Geometry check sheet. Reference: the model listing, model coordinates, mm. Face numbers are marked on the shaded views. A direction names the side the tool comes from. Coordinates: 2 decimals unless noted, no trailing zeros. Write each loop counter-clockwise with the first axis right and the second up, starting at its lowest first coordinate (ties: lowest second). Pieces come first, ordered by that corner, then holes. Notation, with made-up numbers: M 50.25,11 L 106.25,11 A20 cw 106.25,35 Z; hole C -29,72.25 d4. An arc over 180 degrees is marked long. Write each question's results on one line, items separated by ' | '.
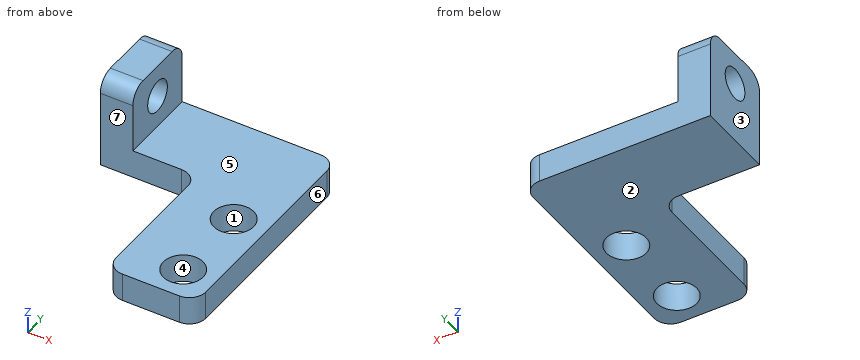
Autodesk Inventor part; units mm, degrees
ref_plane "YZ Plane" through (0, 0, 0) normal (1, 0, 0) x (0, 1, 0)
ref_plane "XZ Plane" through (0, 0, 0) normal (0, 1, 0) x (-1, 0, 0)
ref_plane "XY Plane" through (0, 0, 0) normal (0, 0, 1) x (1, 0, 0)
ref_plane "Work Plane1" through (0, 0, 0) normal (0, 0, 1) x (1, 0, 0)
sketch "Sketch1" plane through (0, 0, 0) normal (0, 0, 1) x (1, 0, 0)
  circle A0 centre (-18.4345, 53.6439) radius 1.95
  circle A1 centre (-18.4345, 43.6439) radius 1.95
  circle A2 centre (-45.5, -14.5) radius 2.1
  circle A3 centre (-14.5, -14.5) radius 2.1
  circle A4 centre (-14.5, 16.5) radius 2.1
  circle A5 centre (-45.5, 16.5) radius 2.1
  circle A6 centre (-30, 1) radius 13
  arc A7 (30, -41.6762) -> (-30, -41.6762) centre (0, -65) ccw
  line L0 (30, -41.6762) -> (30, -22)
  line L1 (30, -22) -> (10.1716, -22)
  line L2 (10.1716, -22) -> (7, -18.8284)
  line L3 (7, -18.8284) -> (7, 20.8284)
  line L4 (7, 20.8284) -> (10.1716, 24)
  line L5 (10.1716, 24) -> (26, 24)
  line L6 (26, 70.5) -> (26, 24)
  arc A8 (26, 70.5) -> (5.5, 91) centre (5.5, 70.5) ccw
  line L7 (-5.5, 91) -> (5.5, 91)
  arc A9 (-5.5, 91) -> (-26, 70.5) centre (-5.5, 70.5) ccw
  line L8 (-26, 24) -> (-26, 70.5)
  line L9 (-26, 24) -> (-49.8284, 24)
  line L10 (-49.8284, 24) -> (-53, 20.8284)
  line L11 (-53, 20.8284) -> (-53, -18.8284)
  line L12 (-53, -18.8284) -> (-49.8284, -22)
  line L13 (-49.8284, -22) -> (-30, -22)
  line L14 (-30, -22) -> (-30, -41.6762)
  circle A10 centre (18.4345, 43.6439) radius 1.95
  circle A11 centre (18.4345, 53.6439) radius 1.95
  line L15 (11.4345, 57.6439) -> (22.4345, 57.6439)
  line L16 (22.4345, 57.6439) -> (22.4345, 39.6439)
  line L17 (22.4345, 39.6439) -> (11.4345, 39.6439)
  line L18 (11.4345, 39.6439) -> (11.4345, 57.6439)
  circle A12 centre (18.4345, 53.6439) radius 2.45
  circle A13 centre (18.4345, 43.6439) radius 2.45
  line L19 (11.4345, 39.6439) -> (11.4345, 57.6439)
  line L20 (11.4345, 57.6439) -> (22.4345, 57.6439)
  line L21 (22.4345, 57.6439) -> (22.4345, 67.6439)
  line L22 (22.4345, 67.6439) -> (11.4345, 67.6439)
  line L23 (11.4345, 67.6439) -> (11.4345, 57.6439)
  line L24 (9.2719, 63.6439) -> (5.8371, 63.6439)
  line L25 (11.4345, 67.6439) -> (-0.5655, 67.6439)
  line L26 (-0.5655, 67.6439) -> (-0.5655, 57.8782)
  line L27 (-0.5655, 57.8782) -> (11.4345, 57.8782)
  line L28 (11.4345, 57.8782) -> (11.4345, 67.6439)
  point P0 (0, 0)
  point P1 (11.4345, 48.6439)
  dimension "d0" = 4
  dimension "d1" = 4
  dimension "d2" = 4
  dimension "d3" = 7
  dimension "d13" = 0.5
  dimension "d14" = 0.5
  dimension "d27" = 15
  dimension "d28" = 4
  dimension "d29" = 11
  dimension "d30" = 12
  dimension "d31" = 90
  dimension "d32" = 79.8782
  dimension "d33" = 61.6439
  dimension "d34" = 20.7281
  dimension "d35" = 24.1629
extrude "Extrusion1" add sketch "Sketch1" along normal blind 3.5 contours L23 L22 L21 L15 | L15 L16 L17 L18 | L27 L26 L25 L23
sketch "Sketch3" plane through (0, 0, 3.5) normal (0, 0, 1) x (1, 0, 0)
  circle A0 centre (18.4345, 43.6439) radius 2.45
  circle A1 centre (18.4345, 53.6439) radius 2.45
  line L0 (11.4345, 39.6439) -> (22.4345, 39.6439)
  line L1 (22.4345, 39.6439) -> (22.4345, 67.6439)
  line L2 (22.4345, 67.6439) -> (-0.5655, 67.6439)
  line L3 (-0.5655, 67.6439) -> (-0.5655, 57.8782)
  line L4 (-0.5655, 57.8782) -> (11.4345, 57.8782)
  line L5 (11.4345, 57.8782) -> (11.4345, 39.6439)
  line L6 (-0.5655, 67.6439) -> (3.4345, 67.6439)
  line L7 (3.4345, 67.6439) -> (3.4345, 57.8782)
  line L8 (3.4345, 57.8782) -> (-0.5655, 57.8782)
  line L9 (-0.5655, 57.8782) -> (-0.5655, 67.6439)
  point P0 (0, 0)
  dimension "d36" = 4
extrude "Extrusion3" add sketch "Sketch3" along normal blind 8 contours L4 L3 L2 L7
sketch "Sketch5" plane through (3.4345, 57.8782, 3.5) normal (1, 0, 0) x (0, 0, -1)
  line L0 (0, 9.7657) -> (0, 0)
  line L1 (0, 9.7657) -> (-8, 9.7657)
  line L2 (-8, 0) -> (-8, 9.7657)
  line L3 (0, 0) -> (-8, 0)
  line L4 (3.5, -18.2343) -> (3.5, 9.7657)
  line L5 (3.5, 9.7657) -> (0, 9.7657)
  line L6 (0, -18.2343) -> (0, 9.7657)
  line L7 (3.5, -18.2343) -> (0, -18.2343)
  circle A0 centre (-4, 4.8829) radius 1.95
  point P0 (3.5, -57.8782)
  dimension "d37" = 3.9
  dimension "d38" = 7.5
extrude "Extrusion5" cut sketch "Sketch5" against normal through all contours A0
fillet "Fillet1" radius 2 6 edges at (22.4345, 39.6439, 1.75) (22.4345, 67.6439, 1.75) (11.4345, 57.8782, 1.75) (11.4345, 39.6439, 1.75) (1.4345, 57.8782, 11.5) (1.4345, 67.6439, 11.5)
properties part number "midle-tensioner_3DPrint"
Q1. Scan lines: probe 1 along Y at (x, z) = (18.5, 2.5); probe 2 along Y at (x, z) = (2.3, 7.5); probe 3 along X at (y, z) = (65.5, 5.25). Record each from-to range of solid material in increasing order.
Geometry check:
probe 1: y = 39.64 to 41.19, 46.09 to 51.19, 56.09 to 67.64 | probe 2: y = 57.88 to 60.81, 64.71 to 67.64 | probe 3: x = -0.57 to 3.43
Q2. Sectioned sample at C-C on y = 52. Record the cut outline in (x, z).
Geometry check:
outline: M 11.43,0 L 16.62,0 L 16.62,3.5 L 11.43,3.5 Z; M 20.25,0 L 22.43,0 L 22.43,3.5 L 20.25,3.5 Z
Q3. Depth check by flat-ended pin: P1, Ø6, axis at y = 62.76, z = 7.5, coming from the -X side; P2, Ø2.5, axis at y = 61.5, z = 9, coming from the +X side; P3, Ø5.5, axis at x = 18.43, y = 43.64, coming from the +Z side; P4, Ø2, axis at x = 7.5, z = 1.5, coming from the -Y side. Enter the tip coordinate at first touch or a pass-through.
Geometry check:
P1: stops at x = -0.57 | P2: stops at x = 3.43 | P3: stops at z = 3.5 | P4: stops at y = 57.88
Q4. Access from +Z, -Z, +X, -X, +Y, -Y to the whole of each face (thin tool, end or side, straight path). Record for the marked faces 5, 6 and 7.
Geometry check:
face 5: +Z, +X, +Y, -Y | face 6: +Z, -Z, +X, +Y, -Y | face 7: +Z, -Z, -X, -Y
Q5. Sectioned sample at B-B on x = 17.5. Record the cut outline in (y, z), and give its area (3 significant figures).
Geometry check:
outline: M 39.64,0 L 41.38,0 L 41.38,3.5 L 39.64,3.5 Z; M 45.91,0 L 51.38,0 L 51.38,3.5 L 45.91,3.5 Z; M 55.91,0 L 67.64,0 L 67.64,3.5 L 55.91,3.5 Z | area: 66.3 mm2
Q6. Sectioned sample at A-A on z = 7.5. Record the cut outline in (x, y), and give its area (3 significant figures).
Geometry check:
outline: M -0.57,57.88 L 3.43,57.88 L 3.43,60.81 L -0.57,60.81 Z; M -0.57,64.71 L 3.43,64.71 L 3.43,67.64 L -0.57,67.64 Z | area: 23.5 mm2
Q7. Sectioned sample at D-D on z = 1.5. Record the cut outline in (x, y).
Geometry check:
outline: M -0.57,57.88 L 9.43,57.88 A2 cw 11.43,55.88 L 11.43,41.64 A2 ccw 13.43,39.64 L 20.43,39.64 A2 ccw 22.43,41.64 L 22.43,65.64 A2 ccw 20.43,67.64 L -0.57,67.64 Z; hole C 18.43,43.64 d4.9; hole C 18.43,53.64 d4.9
Q8. Mould release check, pull along X, two halves, no side actions. Record for the marked faces 1, 2, 3 and 4: pulls with the +X half, pulls with the -X half, needs draft (parallel to the pull), parting line crosses it, or undercut.
Geometry check:
face 1: undercut | face 2: needs draft | face 3: pulls with the -X half | face 4: undercut
